from build123d import *

# Parameters (mm, degrees)
BOSS_EXTRUDE1_DEPTH              = 2
SKETCH2_R                        = 8.9
BOSS_EXTRUDE2_DEPTH              = 2
SKETCH3_R                        = 2
BOSS_EXTRUDE3_DEPTH              = 3
M3_5_CLEARANCE_HOLE1_D           = 3.9
M3_5_CLEARANCE_HOLE1_CSINK_D     = 3.95
M3_5_CLEARANCE_HOLE1_CSINK_ANGLE = 90


with BuildPart() as part:
    # Sketch1 → Boss-Extrude1 (new body)
    with BuildSketch(Plane.XY):
        with BuildLine():
            Line((-10, 0), (-10, -22))
            Line((-10, -22), (10, -22))
            Line((10, -22), (10, 0))
            ThreePointArc((10, 0), (0, 10), (-10, 0))
        make_face()
    extrude(amount=BOSS_EXTRUDE1_DEPTH)

    # Sketch2 → Boss-Extrude2 (add)
    with BuildSketch(Plane(origin=(0, 0, 0), x_dir=(-1, 0, 0), z_dir=(0, 0, -1))):
        Circle(SKETCH2_R)
    extrude(amount=BOSS_EXTRUDE2_DEPTH)

    # Sketch3 → Boss-Extrude3 (add)
    with BuildSketch(Plane(origin=(0, 0, -2), x_dir=(-1, 0, 0), z_dir=(0, 0, -1))):
        Circle(SKETCH3_R)
    extrude(amount=BOSS_EXTRUDE3_DEPTH)

    # M3.5 Clearance Hole1 (through all)
    with Locations(Plane.XY.offset(2)):
        with Locations((-4.784779524, -16.781056018), (4.667291899, -16.141017378)):
            CounterSinkHole(M3_5_CLEARANCE_HOLE1_D / 2, M3_5_CLEARANCE_HOLE1_CSINK_D / 2, counter_sink_angle=M3_5_CLEARANCE_HOLE1_CSINK_ANGLE)


solid = part.part
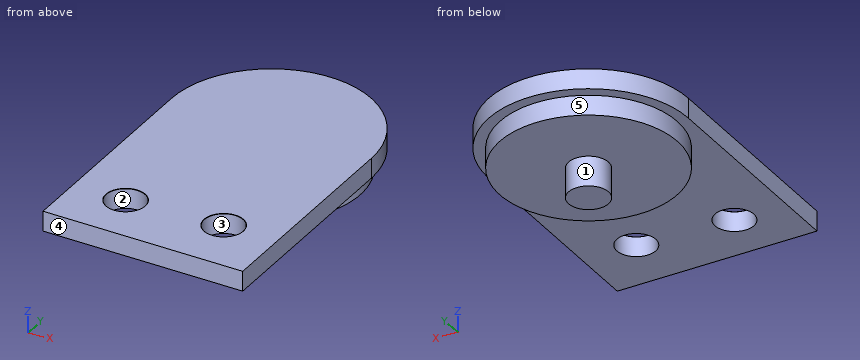
Read the model definition and answer for the solid it produces. Units are mm, in the model's axes. Face numbers are marked on the shaded views. A direction names the side the tool comes from. Round coordinates to 2 decimals unless told otherwise and drop trailing zeros. Write each loop counter-clockwise with the first axis right and the second up, starting at its lowest first coordinate (ties: lowest second). Pieces come first, ordered by that corner, then holes.
1. The part is cut by section D-D, the plane z = -3. Determine the outline of the cut face in (x, y).
2. The part is cut by section C-C, the plane x = -8. Determine the outline of the cut face in (y, z).
3. Given pin 1 Ø3 at (x, y) = (-2.5, -3) entering from -Z; pin 2 Ø6 at (x, y) = (-4.78, -16.78) entering from -Z, each flat-ended and moving along its own axis, determine where each tip first touches the part or whether it passes through.
4. Which of the six approach directions +Z, -Z, +X, -X, +Y, -Y give full straight-line access (tool end or side, diameter ignored) to the marked faces 1 and 2?
5. Straight lines are drawn through the part: L1, parallel to Z at x = 6.75, y = -19; L2, parallel to Z at x = -8.5, y = 0.5; L3, parallel to Y at x = 0, z = 1.5. For each, find the intervals that lie inside material, in ascending order.
6. Determine the mould class of the marked faces 3, 4 and 5 for opening direction Y: pulls with the +Y half, pulls with the -Y half, needs draft (parallel to the pull), parting line crosses it, or undercut.
7. The part is cut by section B-B, the plane y = -6. Determine the outline of the cut face in (x, z).
8. The part is cut by section A-A, the plane x = 0. Determine the outline of the cut face in (y, z), then the cut area to 3 significant figures.
Values:
1. outline: circle Ø4 at (0, 0)
2. outline: (-22, 0) - (-3.9, 0) - (-3.9, -2) - (3.9, -2) - (3.9, 0) - (6, 0) - (6, 2) - (-22, 2) - close
3. pin 1: stops at z = -2
3. pin 2: stops at z = 0
4. face 1: -Z
4. face 2: +Z, -Z
5. L1: z = 0 to 2
5. L2: z = -2 to 2
5. L3: y = -22 to 10
6. face 3: undercut
6. face 4: pulls with the -Y half
6. face 5: parting line crosses it
7. outline: (-10, 0) - (-6.57, 0) - (-6.57, -2) - (6.57, -2) - (6.57, 0) - (10, 0) - (10, 2) - (-10, 2) - close
8. outline: (-22, 0) - (-8.9, 0) - (-8.9, -2) - (-2, -2) - (-2, -5) - (2, -5) - (2, -2) - (8.9, -2) - (8.9, 0) - (10, 0) - (10, 2) - (-22, 2) - close
8. area: 112 mm2
